```python
from build123d import *

# Parameters (mm, degrees)
SKETCH1_W               = 120
SKETCH1_H               = 4
BOSS_EXTRUDE1_DEPTH     = 15
CUT_EXTRUDE1_DEPTH      = 27
CUT_EXTRUDE1_DEPTH_BACK = 130
SKETCH4_R               = 4.5
CUT_EXTRUDE2_DEPTH      = 44


with BuildPart() as part:
    # Sketch1 → Boss-Extrude1 (new body)
    with BuildSketch(Plane.XY):
        with Locations((-39.26849149, 32.447485816)):
            Rectangle(SKETCH1_W, SKETCH1_H)
    extrude(amount=BOSS_EXTRUDE1_DEPTH)

    # Sketch3 → Cut-Extrude1 (cut, two sides)
    with BuildSketch(Plane(origin=(0, 0, 0), x_dir=(0, 0, -1), z_dir=(1, 0, 0))) as cut_extrude1_sk:
        Polygon((-9.5, 30.447485816), (-5.5, 30.447485816), (-5.5, 31.699233238), (-3.5, 31.699233238), (-3.5, 33.429568038), (-11.5, 33.429568038), (-11.5, 31.699233238), (-9.5, 31.699233238), align=None)
    extrude(amount=CUT_EXTRUDE1_DEPTH, mode=Mode.SUBTRACT)
    extrude(cut_extrude1_sk.sketch, amount=-CUT_EXTRUDE1_DEPTH_BACK, mode=Mode.SUBTRACT)

    # Sketch4 → Cut-Extrude2 (cut)
    with BuildSketch(Plane(origin=(0, 0, 0), x_dir=(1, 0, 0), z_dir=(0, 1, 0))):
        with Locations((-39.26849149, -7.5)):
            Circle(SKETCH4_R)
    extrude(amount=CUT_EXTRUDE2_DEPTH, mode=Mode.SUBTRACT)


solid = part.part
```
Check sheet for the modelled part. Datum: model origin and axes. Units: mm. A direction names the side the tool comes from. Round coordinates to 2 decimals unless told otherwise and drop trailing zeros. Write each loop counter-clockwise with the first axis right and the second up, starting at its lowest first coordinate (ties: lowest second). Pieces come first, ordered by that corner, then holes. Notation, with made-up numbers: (79.25, -10.5) -> (133.25, -10.5) arc R22 ccw to (133.25, 1.5) -> close; hole circle Ø7 at (83.25, 44). An arc over 180 degrees is marked (long way). One line per question, with ' | ' between items. Start each with the question number.
1. Sectioned sample at B-B, the plane z = 7.5. Record the cut outline in (x, y), then the cut area to 3 significant figures.
2. Release check for a two-part mould opening along X. For faces 1 (the face through (-43.764, 33.753, 7.302)), 2 (the face through (-40.1, 30.447, 2.7)), 3 (the face through (-99.268, 34, 7)) record: +X half, -X half, draft (parallel to the pull), parting line (faces both ways), or undercut.
3. Sectioned sample at A-A, the plane y = 31.05. Record the cut outline in (x, z), then the cut area to 3 significant figures.
4. Depth check by flat-ended pin: pin 1 (2.5 mm diameter, centred on x = -70, z = 8, fed in from -Y). Enter the tip coordinate at first touch or a pass-through.
5. Scan lines: line 1 along Y through (x, z) = (-20.5, 5.25); line 2 along Z through (x, y) = (-46, 31.3); line 3 along Z through (x, y) = (-18, 31.8). Record each from-to range of solid material in increasing order. Write a range as from..to.
6. Set-up check for faces 4 (the face through (-40, 32, 0)), 5 (the face through (-70, 31.699, 5)): record each of +Z, -Z, +X, -X, +Y, -Y from which the full face is reachable in a straight line by a thin tool's end or side.
7. Sectioned sample at C-C, the plane x = -19.5. Record the cut outline in (y, z), then the cut area to 3 significant figures.
Taken from the geometry:
1) outline: (-99.27, 33.43) -> (-43.77, 33.43) -> (-43.77, 34.45) -> (-99.27, 34.45) -> close; (-34.77, 33.43) -> (20.73, 33.43) -> (20.73, 34.45) -> (-34.77, 34.45) -> close | area: 113 mm^2
2) face 1: undercut | face 2: draft | face 3: -X half
3) outline: (-99.27, 0) -> (20.73, 0) -> (20.73, 5.5) -> (-35.24, 5.5) arc R4.5 cw to (-43.3, 5.5) -> (-99.27, 5.5) -> close; (-99.27, 9.5) -> (-43.3, 9.5) arc R4.5 cw to (-35.24, 9.5) -> (20.73, 9.5) -> (20.73, 15) -> (-99.27, 15) -> close | area: 1,290 mm^2
4) pin 1: stops at y = 33.43
5) line 1: y = 30.45..31.7, 33.43..34.45 | line 2: z = 0..5.5, 9.5..15 | line 3: z = 0..3.5, 11.5..15
6) face 4: -Z, +X, -X, +Y, -Y | face 5: +X, -X
7) outline: (30.45, 0) -> (34.45, 0) -> (34.45, 15) -> (30.45, 15) -> (30.45, 9.5) -> (31.7, 9.5) -> (31.7, 11.5) -> (33.43, 11.5) -> (33.43, 3.5) -> (31.7, 3.5) -> (31.7, 5.5) -> (30.45, 5.5) -> close | area: 41.2 mm^2
